CAD build for the part. Positions are in the model's coordinates, mm. Face numbers are marked on the shaded views. A direction names the side the tool comes from. Coordinates: 2 decimals unless noted, no trailing zeros. Order: outer loops, then holes, each group sorted by start corner. A loop starts at its lowest first (then second) coordinate and runs counter-clockwise, first axis right, second up.
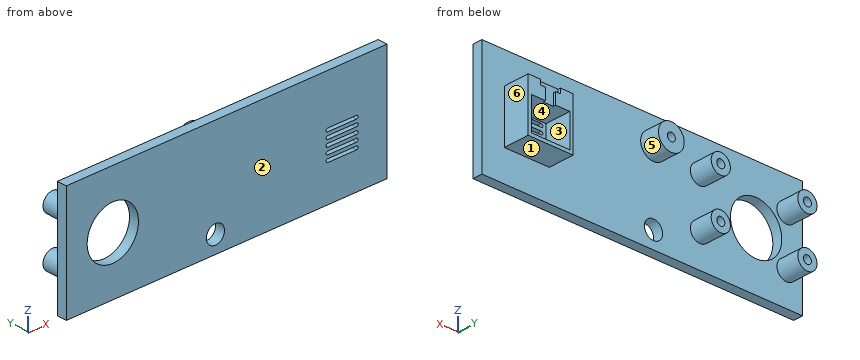
from build123d import *

# Parameters (mm, degrees)
SKETCH1_W           = 100
SKETCH1_H           = 35
BOSS_EXTRUDE1_DEPTH = 3
SKETCH2_R           = 3
BOSS_EXTRUDE2_DEPTH = 7
CUT_EXTRUDE2_REACH  = 108.179
SKETCH3_R           = 8
SKETCH4_R           = 1.25
CUT_EXTRUDE3_DEPTH  = 6
SKETCH5_R           = 4
SKETCH5_R_2         = 1.25
BOSS_EXTRUDE3_DEPTH = 6
CUT_EXTRUDE4_REACH  = 108.419
SKETCH6_R           = 2.83
SKETCH8_W           = 14
SKETCH8_H           = 16
SKETCH8_W_2         = 12
SKETCH8_H_2         = 10
BOSS_EXTRUDE4_DEPTH = 8
CUT_EXTRUDE5_DEPTH  = 0.8
CUT_EXTRUDE6_REACH  = 108.25


with BuildPart() as part:
    # Sketch1 → Boss-Extrude1 (new body)
    with BuildSketch(Plane(origin=(0, 0, 0), x_dir=(1, 0, 0), z_dir=(0, 1, 0))):
        with Locations((50, 17.5)):
            Rectangle(SKETCH1_W, SKETCH1_H)
    extrude(amount=BOSS_EXTRUDE1_DEPTH)

    # Sketch2 → Boss-Extrude2 (add)
    with BuildSketch(Plane(origin=(0, 3, 0), x_dir=(1, 0, 0), z_dir=(0, 1, 0))):
        with Locations(Location((5, 25, 0), (0, 0, 90))):
            Circle(SKETCH2_R)
        with Locations(Location((5, 10, 0), (0, 0, 90))):
            Circle(SKETCH2_R)
        with Locations(Location((32, 10, 0), (0, 0, 90))):
            Circle(SKETCH2_R)
        with Locations(Location((32, 25, 0), (0, 0, 90))):
            Circle(SKETCH2_R)
    extrude(amount=BOSS_EXTRUDE2_DEPTH)

    # Sketch3 → Cut-Extrude2 (cut, up to next)
    with BuildSketch(Plane(origin=(0, 3, 0), x_dir=(1, 0, 0), z_dir=(0, 1, 0)), mode=Mode.PRIVATE) as cut_extrude2_sk1:
        with Locations(Location((14.5, 17.5, 0), (0, 0, 270))):
            Circle(SKETCH3_R)
    cut_extrude2_tool1 = extrude(cut_extrude2_sk1.sketch, amount=-CUT_EXTRUDE2_REACH, mode=Mode.PRIVATE) & part.part
    add(cut_extrude2_tool1.solids().sort_by_distance((14.5, 3, -17.5))[0], mode=Mode.SUBTRACT)

    # Sketch4 → Cut-Extrude3 (cut)
    with BuildSketch(Plane(origin=(0, 10, 0), x_dir=(1, 0, 0), z_dir=(0, 1, 0))):
        with Locations(Location((32, 25, 0), (0, 0, 270))):
            Circle(SKETCH4_R)
        with Locations(Location((32, 10, 0), (0, 0, 270))):
            Circle(SKETCH4_R)
        with Locations(Location((5, 10, 0), (0, 0, 270))):
            Circle(SKETCH4_R)
        with Locations(Location((5, 25, 0), (0, 0, 270))):
            Circle(SKETCH4_R)
    extrude(amount=-CUT_EXTRUDE3_DEPTH, mode=Mode.SUBTRACT)

    # Sketch5 → Boss-Extrude3 (add)
    with BuildSketch(Plane(origin=(0, 3, 0), x_dir=(1, 0, 0), z_dir=(0, 1, 0))):
        with Locations(Location((46.5, 8, 0), (0, 0, 90))):
            Circle(SKETCH5_R)
        with Locations(Location((46.5, 8, 0), (0, 0, 270))):
            Circle(SKETCH5_R_2, mode=Mode.SUBTRACT)
    extrude(amount=BOSS_EXTRUDE3_DEPTH)

    # Sketch6 → Cut-Extrude4 (cut, up to next)
    with BuildSketch(Plane.XZ, mode=Mode.PRIVATE) as cut_extrude4_sk1:
        with Locations(Location((46.5, -29.75, 0), (0, 0, 270))):
            Circle(SKETCH6_R)
    cut_extrude4_tool1 = extrude(cut_extrude4_sk1.sketch, amount=-CUT_EXTRUDE4_REACH, mode=Mode.PRIVATE) & part.part
    add(cut_extrude4_tool1.solids().sort_by_distance((46.5, 0, -29.75))[0], mode=Mode.SUBTRACT)

    # Sketch8 → Boss-Extrude4 (add)
    with BuildSketch(Plane(origin=(0, 3, 0), x_dir=(1, 0, 0), z_dir=(0, 1, 0))):
        with Locations((86, 17.5)):
            Rectangle(SKETCH8_W, SKETCH8_H)
        with Locations((86, 19.5)):
            Rectangle(SKETCH8_W_2, SKETCH8_H_2, mode=Mode.SUBTRACT)
    extrude(amount=BOSS_EXTRUDE4_DEPTH)

    # Sketch9 → Cut-Extrude5 (cut)
    with BuildSketch(Plane(origin=(0, 11, 0), x_dir=(1, 0, 0), z_dir=(0, 1, 0))):
        Polygon((84.4, 14.5), (84.4, 11), (82.9, 11), (82.9, 9.5), (89.1, 9.5), (89.1, 11), (87.6, 11), (87.6, 14.5), align=None)
    extrude(amount=-CUT_EXTRUDE5_DEPTH, mode=Mode.SUBTRACT)

    # Sketch10 → Cut-Extrude6 (cut, up to next)
    with BuildSketch(Plane(origin=(0, 3, 0), x_dir=(1, 0, 0), z_dir=(0, 1, 0)), mode=Mode.PRIVATE) as cut_extrude6_sk1:
        with BuildLine():
            Line((81.5, 24), (90.5, 24))
            ThreePointArc((90.5, 24), (91, 23.5), (90.5, 23))
            Line((90.5, 23), (81.5, 23))
            ThreePointArc((81.5, 23), (81, 23.5), (81.5, 24))
        make_face()
    cut_extrude6_tool1 = extrude(cut_extrude6_sk1.sketch, amount=-CUT_EXTRUDE6_REACH, mode=Mode.PRIVATE) & part.part
    # Sketch10 → Cut-Extrude6 (cut, up to next)
    with BuildSketch(Plane(origin=(0, 3, 0), x_dir=(1, 0, 0), z_dir=(0, 1, 0)), mode=Mode.PRIVATE) as cut_extrude6_sk2:
        with BuildLine():
            Line((81.5, 22), (90.5, 22))
            ThreePointArc((90.5, 22), (91, 21.5), (90.5, 21))
            Line((90.5, 21), (81.5, 21))
            ThreePointArc((81.5, 21), (81, 21.5), (81.5, 22))
        make_face()
    cut_extrude6_tool2 = extrude(cut_extrude6_sk2.sketch, amount=-CUT_EXTRUDE6_REACH, mode=Mode.PRIVATE) & part.part
    # Sketch10 → Cut-Extrude6 (cut, up to next)
    with BuildSketch(Plane(origin=(0, 3, 0), x_dir=(1, 0, 0), z_dir=(0, 1, 0)), mode=Mode.PRIVATE) as cut_extrude6_sk3:
        with BuildLine():
            Line((81.5, 20), (90.5, 20))
            ThreePointArc((90.5, 20), (91, 19.5), (90.5, 19))
            Line((90.5, 19), (81.5, 19))
            ThreePointArc((81.5, 19), (81, 19.5), (81.5, 20))
        make_face()
    cut_extrude6_tool3 = extrude(cut_extrude6_sk3.sketch, amount=-CUT_EXTRUDE6_REACH, mode=Mode.PRIVATE) & part.part
    # Sketch10 → Cut-Extrude6 (cut, up to next)
    with BuildSketch(Plane(origin=(0, 3, 0), x_dir=(1, 0, 0), z_dir=(0, 1, 0)), mode=Mode.PRIVATE) as cut_extrude6_sk4:
        with BuildLine():
            Line((81.5, 18), (90.5, 18))
            ThreePointArc((90.5, 18), (91, 17.5), (90.5, 17))
            Line((90.5, 17), (81.5, 17))
            ThreePointArc((81.5, 17), (81, 17.5), (81.5, 18))
        make_face()
    cut_extrude6_tool4 = extrude(cut_extrude6_sk4.sketch, amount=-CUT_EXTRUDE6_REACH, mode=Mode.PRIVATE) & part.part
    # Sketch10 → Cut-Extrude6 (cut, up to next)
    with BuildSketch(Plane(origin=(0, 3, 0), x_dir=(1, 0, 0), z_dir=(0, 1, 0)), mode=Mode.PRIVATE) as cut_extrude6_sk5:
        with BuildLine():
            Line((81.5, 16), (90.5, 16))
            ThreePointArc((90.5, 16), (91, 15.5), (90.5, 15))
            Line((90.5, 15), (81.5, 15))
            ThreePointArc((81.5, 15), (81, 15.5), (81.5, 16))
        make_face()
    cut_extrude6_tool5 = extrude(cut_extrude6_sk5.sketch, amount=-CUT_EXTRUDE6_REACH, mode=Mode.PRIVATE) & part.part
    add(cut_extrude6_tool1.solids().sort_by_distance((86, 3, -23.5))[0], mode=Mode.SUBTRACT)
    add(cut_extrude6_tool2.solids().sort_by_distance((86, 3, -21.5))[0], mode=Mode.SUBTRACT)
    add(cut_extrude6_tool3.solids().sort_by_distance((86, 3, -19.5))[0], mode=Mode.SUBTRACT)
    add(cut_extrude6_tool4.solids().sort_by_distance((86, 3, -17.5))[0], mode=Mode.SUBTRACT)
    add(cut_extrude6_tool5.solids().sort_by_distance((86, 3, -15.5))[0], mode=Mode.SUBTRACT)


solid = part.part
1) Pin check, flat tips, straight feed: P1, Ø3, axis at x = 32, z = -10, coming from the +Y side; P2, Ø2, axis at x = 13.5, z = -31, coming from the -Y side; P3, Ø1.2, axis at x = 46.5, z = -8, coming from the +Y side; P4, Ø0.6, axis at y = 10.5, z = -10.5, coming from the +X side. Stop position of each tip, or through.
2) Slice it at A-A (y = 6). Give the number of separate pieces and of enclosed holes in the cut face, plus the area to 3 significant figures.
3) Which spindle directions (+Z, -Z, +X, -X, +Y, -Y) get a long thin tool onto all of the face, cutting with end or side? Do the marked faces 1, 2 and 3. Say none if no direction does.
4) Slice it at D-D (x = 32). List the corners of the cut face in (y, z), plus the area to 3 significant figures.
5) Slice it at C-C (x = 46.5). List the corners of the cut face in (y, z), plus the area to 3 significant figures.
6) Slice it at B-B (z = -29.75). List the corners of the cut face in (x, y), plus the area to 3 significant figures.
7) Drill centre lines: probe 1 along X at (y, z) = (1.05, -17.5); probe 2 along X at (y, z) = (3.5, -18); probe 3 along X at (y, z) = (5.55, -25). Where is each one in solid material? Low to high.
8) Two-plate mould, pull along Z, no slides. Class the marked faces 4, 5 and 6: released by +Z, released by -Z, zero draft, split by the parting line, or undercut.
Worked out:
1. P1: stops at y = 10
1. P2: stops at y = 0
1. P3: stops at y = 3
1. P4: stops at x = 93
2. separate pieces: 6
2. enclosed holes: 6
2. area: 243 mm2
3. face 1: -Z, +X, +Y
3. face 2: +Z, -Z, +X, -X, -Y
3. face 3: +Y
4. outline: (0, -35) - (3, -35) - (3, -28) - (10, -28) - (10, -26.25) - (4, -26.25) - (4, -23.75) - (10, -23.75) - (10, -22) - (3, -22) - (3, -13) - (10, -13) - (10, -11.25) - (4, -11.25) - (4, -8.75) - (10, -8.75) - (10, -7) - (3, -7) - (3, 0) - (0, 0) - close
4. area: 159 mm2
5. outline: (0, -35) - (3, -35) - (3, -32.58) - (0, -32.58) - close; (0, -26.92) - (3, -26.92) - (3, -12) - (9, -12) - (9, -9.25) - (3, -9.25) - (3, -6.75) - (9, -6.75) - (9, -4) - (3, -4) - (3, 0) - (0, 0) - close
5. area: 121 mm2
6. outline: (0, 0) - (43.67, 0) - (43.67, 3) - (0, 3) - close; (49.33, 0) - (100, 0) - (100, 3) - (49.33, 3) - close
6. area: 283 mm2
7. probe 1: x = 0 to 6.5, 22.5 to 81, 91 to 100
7. probe 2: x = 79 to 80, 92 to 93
7. probe 3: x = 2 to 3.75, 6.25 to 8, 29 to 30.75, 33.25 to 35, 79 to 93
8. face 4: undercut
8. face 5: split by the parting line
8. face 6: zero draft
